Check sheet for the modelled part. Datum: model origin and axes. Units: mm. Give positions to 0.01 mm unless a question says otherwise; leave off trailing zeros. Order: outer loops, then holes, each group sorted by start corner. A loop starts at its lowest first (then second) coordinate and runs counter-clockwise, first axis right, second up. Notation, with made-up numbers: (-17, 73) - (16, 73) arc R8 ccw to (16, 77) - close; hole circle Ø11 at (37, 41). An arc over 180 degrees is marked (long way). Answer in a Markdown table with one row per item.
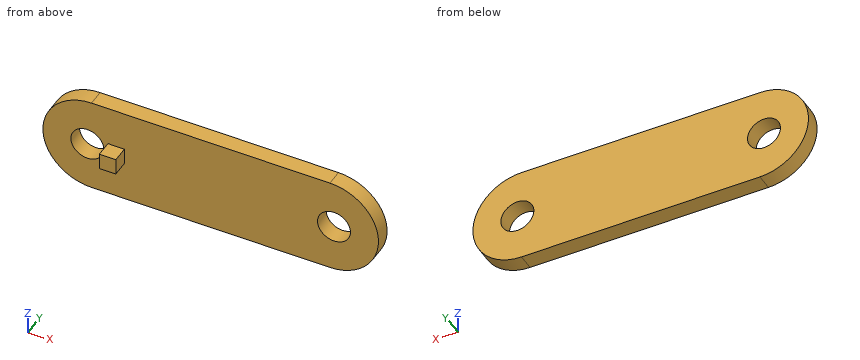
from build123d import *

# Parameters (mm, degrees)
BOSS_EXTRUDE1_DEPTH = 2
SKETCH5_R           = 2
CUT_EXTRUDE1_DEPTH  = 76.301439031
SKETCH6_W           = 2
SKETCH6_H           = 2
BOSS_EXTRUDE2_DEPTH = 2


with BuildPart() as part:
    # Sketch4 → Boss-Extrude1 (new body)
    with BuildSketch(Plane(origin=(0, 0, 0), x_dir=(1, 0, 0), z_dir=(0, 1, 0))):
        with BuildLine():
            Line((-69.143298969, 5.9), (-40.200862119, 5.9))
            ThreePointArc((-40.200862119, 5.9), (-34.300862119, 0), (-40.200862119, -5.9))
            Line((-40.200862119, -5.9), (-69.143298969, -5.9))
            ThreePointArc((-69.143298969, -5.9), (-75.043298969, 0), (-69.143298969, 5.9))
        make_face()
    extrude(amount=BOSS_EXTRUDE1_DEPTH)

    # Sketch5 → Cut-Extrude1 (cut, through all)
    with BuildSketch(Plane.XZ):
        with Locations(Location((-39.700862119, 0, 0), (0, 0, 270))):
            Circle(SKETCH5_R)
        with Locations(Location((-69.643298969, 0, 0), (0, 0, 270))):
            Circle(SKETCH5_R)
    extrude(amount=-CUT_EXTRUDE1_DEPTH, mode=Mode.SUBTRACT)

    # Sketch6 → Boss-Extrude2 (add)
    with BuildSketch(Plane.XZ):
        with Locations((-66.143298969, 0)):
            Rectangle(SKETCH6_W, SKETCH6_H)
    extrude(amount=BOSS_EXTRUDE2_DEPTH)


solid = part.part
(1) Cross-section at B-B, the plane z = 1.5. Record the cut outline in (x, y).
Geometry says:
| item | result |
|---|---|
| outline | (-74.85, 0) - (-70.97, 0) - (-70.97, 2) - (-74.85, 2) - close; (-68.32, 0) - (-41.02, 0) - (-41.02, 2) - (-68.32, 2) - close; (-38.38, 0) - (-34.49, 0) - (-34.49, 2) - (-38.38, 2) - close |
(2) Gauge pin test, flat ends, axial feed: P1, Ø0.6, axis at x = -66, y = -1.5, coming from the +Z side; P2, Ø3.5, axis at x = -46.5, z = -3, coming from the -Y side; P3, Ø0.6, axis at y = -1, z = 0.5, coming from the -X side. Record the tip position at first contact, or that the pin passes through.
Geometry says:
| item | result |
|---|---|
| P1 | z = 1 |
| P2 | y = 0 |
| P3 | x = -67.14 |
(3) Cross-section at D-D, the plane x = -57.5. Record the cut outline in (y, z), then the cut area to 3 significant figures.
Geometry says:
| item | result |
|---|---|
| outline | (0, -5.9) - (2, -5.9) - (2, 5.9) - (0, 5.9) - close |
| area | 23.6 mm² |
(4) Cross-section at A-A, the plane z = 0. Record the cut outline in (x, y).
Geometry says:
| item | result |
|---|---|
| outline | (-75.04, 0) - (-71.64, 0) - (-71.64, 2) - (-75.04, 2) - close; (-67.64, 0) - (-67.14, 0) - (-67.14, -2) - (-65.14, -2) - (-65.14, 0) - (-41.7, 0) - (-41.7, 2) - (-67.64, 2) - close; (-37.7, 0) - (-34.3, 0) - (-34.3, 2) - (-37.7, 2) - close |
(5) Cross-section at C-C, the plane y = 0.65. Record the cut outline in (x, z).
Geometry says:
| item | result |
|---|---|
| outline | (-69.14, -5.9) - (-40.2, -5.9) arc R5.9 ccw to (-40.2, 5.9) - (-69.14, 5.9) arc R5.9 ccw to start; hole circle Ø4 at (-69.64, 0); hole circle Ø4 at (-39.7, 0) |
(6) Thickness scan on L1, parallel to X at y = 0.75, z = 0; L2, parallel to X at y = 1.1, z = -0.25; L3, parallel to Y at x = -35.5, z = -1.25. Record the ranges inside material, lowest first.
Geometry says:
| item | result |
|---|---|
| L1 | -75.04 to -71.64, -67.64 to -41.7, -37.7 to -34.3 |
| L2 | -75.04 to -71.63, -67.66 to -41.69, -37.72 to -34.31 |
| L3 | 0 to 2 |
